```python
from build123d import *

# Parameters (mm, degrees)
SKETCH_1_W               = 90
SKETCH_1_H               = 72
EXTRUDE_1_DEPTH          = 25
SKETCH_2_W               = 85.5
SKETCH_2_H               = 32.5
CUT_EXTRUDE_1_DEPTH      = 20
SKETCH_3_W               = 10
SKETCH_3_H               = 20
CUT_EXTRUDE_2_DEPTH      = 1
CUT_EXTRUDE_2_DEPTH_BACK = 91
SKETCH_4_R               = 1.65
CUT_EXTRUDE_3_DEPTH      = 21
CUT_EXTRUDE_3_DEPTH_BACK = 6
SKETCH_5_R               = 3.5
CUT_EXTRUDE_4_DEPTH      = 1
CUT_EXTRUDE_4_DEPTH_BACK = 26


with BuildPart() as part:
    # 草图1 → 凸台-拉伸1 (new body)
    with BuildSketch(Plane.XY):
        Rectangle(SKETCH_1_W, SKETCH_1_H)
    extrude(amount=EXTRUDE_1_DEPTH)

    # 草图2 → 切除-拉伸1 (cut)
    with BuildSketch(Plane.XY.offset(25)):
        with Locations((0, 17.5)):
            Rectangle(SKETCH_2_W, SKETCH_2_H)
        with Locations((0, -17.5)):
            Rectangle(SKETCH_2_W, SKETCH_2_H)
    extrude(amount=-CUT_EXTRUDE_1_DEPTH, mode=Mode.SUBTRACT)

    # 草图3 → 切除-拉伸2 (cut, two sides)
    with BuildSketch(Plane(origin=(45, 0, 0), x_dir=(0, 0, -1), z_dir=(1, 0, 0))) as cut_extrude_2_sk:
        with Locations((-12.5, 17.5)):
            Rectangle(SKETCH_3_W, SKETCH_3_H)
        with Locations((-12.5, -17.5)):
            Rectangle(SKETCH_3_W, SKETCH_3_H)
    extrude(amount=CUT_EXTRUDE_2_DEPTH, mode=Mode.SUBTRACT)
    extrude(cut_extrude_2_sk.sketch, amount=-CUT_EXTRUDE_2_DEPTH_BACK, mode=Mode.SUBTRACT)

    # 草图4 → 切除-拉伸3 (cut, two sides)
    with BuildSketch(Plane.XY.offset(5)) as cut_extrude_3_sk:
        with Locations((-39, 4.5)):
            Circle(SKETCH_4_R)
        with Locations((-39, 30.5)):
            Circle(SKETCH_4_R)
        with Locations((-39, -4.5)):
            Circle(SKETCH_4_R)
        with Locations((-39, -30.5)):
            Circle(SKETCH_4_R)
        with Locations((39, -30.5)):
            Circle(SKETCH_4_R)
        with Locations((39, -4.5)):
            Circle(SKETCH_4_R)
        with Locations((39, 4.5)):
            Circle(SKETCH_4_R)
        with Locations((39, 30.5)):
            Circle(SKETCH_4_R)
    extrude(amount=CUT_EXTRUDE_3_DEPTH, mode=Mode.SUBTRACT)
    extrude(cut_extrude_3_sk.sketch, amount=-CUT_EXTRUDE_3_DEPTH_BACK, mode=Mode.SUBTRACT)

    # 草图5 → 切除-拉伸4 (cut, two sides)
    with BuildSketch(Plane(origin=(0, 0, 0), x_dir=(-1, 0, 0), z_dir=(0, 0, -1))) as cut_extrude_4_sk:
        with Locations((-37.7, 18.8)):
            Circle(SKETCH_5_R)
    extrude(amount=CUT_EXTRUDE_4_DEPTH, mode=Mode.SUBTRACT)
    extrude(cut_extrude_4_sk.sketch, amount=-CUT_EXTRUDE_4_DEPTH_BACK, mode=Mode.SUBTRACT)


solid = part.part
```
Input: part model. Units: mm. Frame: model coordinates. A direction names the side the tool comes from. Coordinates: 2 decimals unless noted, no trailing zeros. Write each loop counter-clockwise with the first axis right and the second up, starting at its lowest first coordinate (ties: lowest second). Pieces come first, ordered by that corner, then holes. Notation, with made-up numbers: (46.25, 73.25) - (104.25, 73.25) arc R25 cw to (104.25, 89.25) - close; hole circle Ø2 at (63.25, 56.25). An arc over 180 degrees is marked (long way). Put each result on its own line as item: value. Start each with the question number.
1) Cut plane D-D (z = 14). Return the cut outline in (x, y).
2) Cut plane C-C (y = 18.8). Return the cut outline in (x, z), plus the area to 3 significant figures.
3) Mould query, pull axis Z, two halves, no side actions, for faces 4 (the face through (38.785, -28.864, 2.535)), 5 (the face through (44, -18, 7.5)), 6 (the face through (-1, -17, 5)). Classes: pulls with the +Z half, pulls with the -Z half, needs draft (parallel to the pull), parting line crosses it, or undercut.
4) Cut plane A-A (y = 4.5). Return the cut outline in (x, z), plus the area to 3 significant figures.
5) Contact query for a flat-ended pin moving along its axis: pin 1 (4 mm diameter, centred on x = 39, y = 4.5, fed in from +Z). Output: stop coordinate, or through.
6) Cut plane B-B (z = 23). Return the cut outline in (x, y), plus the area to 4 significant figures.
7) Ray query, L1, parallel to Y at x = 31.5, z = 14; L2, parallel to Y at x = -39, z = 2.7; L3, parallel to X at y = -16, z = 6.5. Return the intervals inside material, ascending.
8) Reachability of faces 1 (the face through (-42.75, 17, 20)), 2 (the face through (-44, 17, 17.5)), 3 (the face through (37.35, 4.57, 2.54)) from +Z, -Z, +X, -X, +Y, -Y: full face, straight path, thin tool, end or side. Return the list, or none.
Resolved:
1. outline: (-45, -36) - (45, -36) - (45, -27.5) - (42.75, -27.5) - (42.75, -33.75) - (-42.75, -33.75) - (-42.75, -27.5) - (-45, -27.5) - close; (-45, -7.5) - (-42.75, -7.5) - (-42.75, -1.25) - (42.75, -1.25) - (42.75, -7.5) - (45, -7.5) - (45, 7.5) - (42.75, 7.5) - (42.75, 1.25) - (-42.75, 1.25) - (-42.75, 7.5) - (-45, 7.5) - close; (-45, 27.5) - (-42.75, 27.5) - (-42.75, 33.75) - (42.75, 33.75) - (42.75, 27.5) - (45, 27.5) - (45, 36) - (-45, 36) - close
2. outline: (-45, 0) - (34.2, 0) - (34.2, 5) - (-42.75, 5) - (-42.75, 7.5) - (-45, 7.5) - close; (-45, 17.5) - (-42.75, 17.5) - (-42.75, 25) - (-45, 25) - close; (41.2, 0) - (45, 0) - (45, 7.5) - (42.75, 7.5) - (42.75, 5) - (41.2, 5) - close; (42.75, 17.5) - (45, 17.5) - (45, 25) - (42.75, 25) - close
2. area: 460 mm2
3. face 4: needs draft
3. face 5: undercut
3. face 6: pulls with the +Z half
4. outline: (-45, 0) - (-40.65, 0) - (-40.65, 5) - (-42.75, 5) - (-42.75, 25) - (-45, 25) - close; (-37.35, 0) - (37.35, 0) - (37.35, 5) - (-37.35, 5) - close; (40.65, 0) - (45, 0) - (45, 25) - (42.75, 25) - (42.75, 5) - (40.65, 5) - close
4. area: 507 mm2
5. pin 1: stops at z = 5
6. outline: (-45, -36) - (45, -36) - (45, 36) - (-45, 36) - close; hole (-42.75, -33.75) - (42.75, -33.75) - (42.75, -1.25) - (-42.75, -1.25) - close; hole (-42.75, 1.25) - (42.75, 1.25) - (42.75, 33.75) - (-42.75, 33.75) - close
6. area: 922.5 mm2
7. L1: y = -36 to -33.75, -1.25 to 1.25, 33.75 to 36
7. L2: y = -36 to -32.15, -28.85 to -6.15, -2.85 to 2.85, 6.15 to 28.85, 32.15 to 36
7. L3: x = -45 to -42.75, 42.75 to 45
8. face 1: +Z
8. face 2: +X, -X
8. face 3: +Z, -Z
